Verification items for the finished model (mm, model axes). Face numbers are marked on the shaded views. A direction names the side the tool comes from. Round coordinates to 2 decimals unless told otherwise and drop trailing zeros. Write each loop counter-clockwise with the first axis right and the second up, starting at its lowest first coordinate (ties: lowest second). Pieces come first, ordered by that corner, then holes. Notation, with made-up numbers: M 44,-19 L 78,-19 A14 cw 78,7 Z; hole C 8,60.25 d10. An arc over 180 degrees is marked long. One line per item, written item: value. Start each with the question number.
Item 1: Draft check along Z on the marked faces 3, 4 and 5. Enter one of: +Z half, -Z half, draft (parallel to the pull), parting line (faces both ways), or undercut.
Item 2: Section check D-D, the plane z = -5.5. Record the cut outline in (x, y).
Item 3: Section check A-A, the plane x = 0. Record the cut outline in (y, z).
Item 4: Section check B-B, the plane z = 0. Record the cut outline in (x, y), then the cut area to 3 significant figures.
Item 5: Tool access check on the marked faces 1 and 2. Record the directions out of +Z, -Z, +X, -X, +Y, -Y that give a thin tool (end or side, any length) a straight path to the whole face; none if there is none.
Item 6: Section check C-C, the plane y = -4.75. Record the cut outline in (x, z).
Item 7: Gauge pin test, flat ends, axial feed: pin 1 (2 mm diameter, centred on x = -7, z = 6, fed in from -Y); pin 2 (5 mm diameter, centred on x = 0, z = 0, fed in from -Y); pin 3 (6 mm diameter, centred on x = -4.5, y = 7, fed in from +Z); pin 4 (6 mm diameter, centred on y = 1.5, z = -4, fed in from -X). Record the tip position at first contact, or that the pin passes through.
Item 8: Thickness scan on probe 1 along X at (y, z) = (3.5, 0); probe 2 along X at (y, z) = (-9.5, 0); probe 3 along Y at (x, z) = (-7, -4.75). Record the ranges inside material, lowest first. Write a range as from..to.
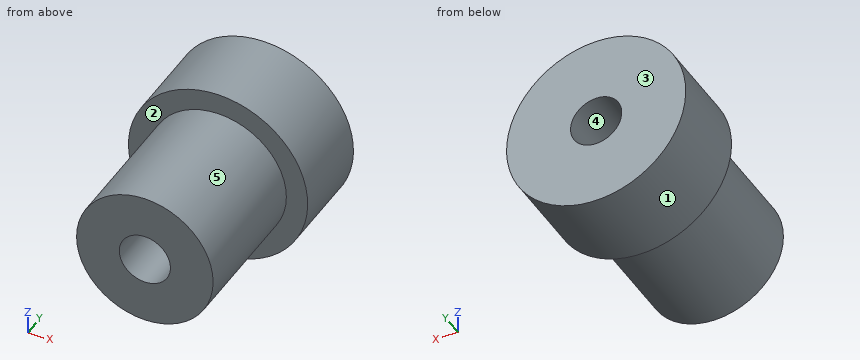
from build123d import *

# Parameters (mm, degrees)
SKETCH1_R               = 10.5
BOSS_EXTRUDE1_DEPTH     = 10
SKETCH2_R               = 8
BOSS_EXTRUDE2_DEPTH     = 16
CUT_EXTRUDE1_DEPTH      = 22.828879953
CUT_EXTRUDE1_DEPTH_BACK = 22.828879953
SKETCH3_R               = 3


with BuildPart() as part:
    # Sketch1 → Boss-Extrude1 (new body)
    with BuildSketch(Plane(origin=(0, 0, 0), x_dir=(1, 0, 0), z_dir=(0, 1, 0))):
        with Locations(Location((0, 0, 0), (0, 0, 270))):
            Circle(SKETCH1_R)
    extrude(amount=BOSS_EXTRUDE1_DEPTH)

    # Sketch2 → Boss-Extrude2 (add)
    with BuildSketch(Plane(origin=(0, 0, 0), x_dir=(1, 0, 0), z_dir=(0, 1, 0))):
        with Locations(Location((0, 0, 0), (0, 0, 270))):
            Circle(SKETCH2_R)
    extrude(amount=-BOSS_EXTRUDE2_DEPTH)

    # Sketch3 → Cut-Extrude1 (cut, two sides: drawn at the far end of the back side and taken through both)
    with BuildSketch(Plane(origin=(0, 0, 0), x_dir=(1, 0, 0), z_dir=(0, 1, 0)).offset(-CUT_EXTRUDE1_DEPTH_BACK)):
        with Locations(Location((0, 0, 0), (0, 0, 270))):
            Circle(SKETCH3_R)
    extrude(amount=CUT_EXTRUDE1_DEPTH + CUT_EXTRUDE1_DEPTH_BACK, mode=Mode.SUBTRACT)


solid = part.part
Response values:
1. face 3: draft
1. face 4: undercut
1. face 5: parting line
2. outline: M -8.94,0 L -5.81,0 L -5.81,-16 L 5.81,-16 L 5.81,0 L 8.94,0 L 8.94,10 L -8.94,10 Z
3. outline: M -16,-8 L 0,-8 L 0,-10.5 L 10,-10.5 L 10,-3 L -16,-3 Z; M -16,3 L 10,3 L 10,10.5 L 0,10.5 L 0,8 L -16,8 Z
4. outline: M -10.5,0 L -8,0 L -8,-16 L -3,-16 L -3,10 L -10.5,10 Z; M 3,-16 L 8,-16 L 8,0 L 10.5,0 L 10.5,10 L 3,10 Z
4. area: 310 mm2
5. face 1: +Y, -Y
5. face 2: -Y
6. outline: C 0,0 d16; hole C 0,0 d6
7. pin 1: stops at y = 0
7. pin 2: passes through
7. pin 3: stops at z = 10.39
7. pin 4: stops at x = -10.45
8. probe 1: x = -10.5..-3, 3..10.5
8. probe 2: x = -8..-3, 3..8
8. probe 3: y = 0..10
